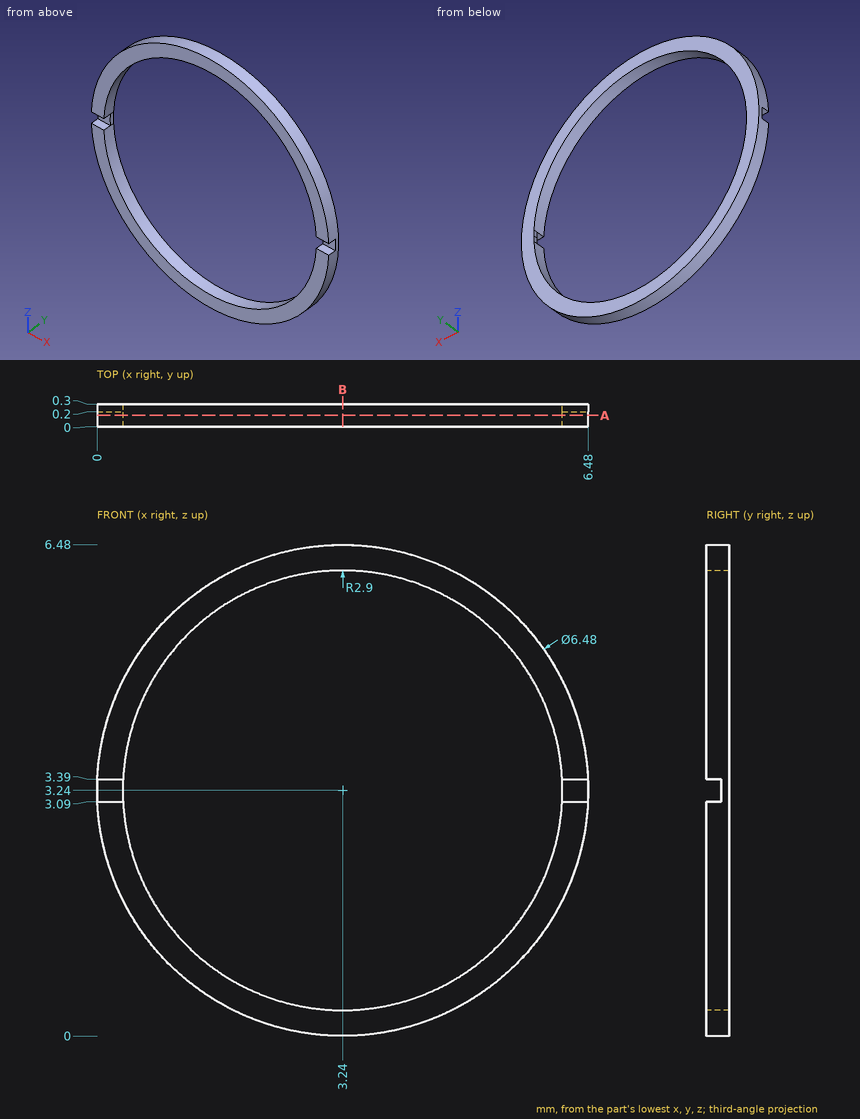
Could you check a few things on this drawing? It's one solid part, dimensions in mm from its lowest x, y, z. Round coordinates to 2 decimals unless told otherwise and drop trailing zeros. Write each loop counter-clockwise with the first axis right and the second up, starting at its lowest first coordinate (ties: lowest second). Pieces come first, ordered by that corner, then holes.
Q1. If we section it at A-A on y = 0.15: Write out the boundary of the cut face in (x, z).
Q2. If we section it at B-B on x = 3.24: Write out the boundary of the cut face in (y, z).
Q3. Please list where these lines run through material, in increasing order: probe 1 along Z at (x, y) = (4.25, 0.15); probe 2 along X at (y, z) = (0.2, 3.75); probe 3 along X at (y, z) = (0.2, 3.5).
Answer below:
1. outline: (0, 3.09) arc R3.24 ccw to (6.48, 3.09) - (6.14, 3.09) arc R2.9 cw to (0.34, 3.09) - close; (0, 3.39) - (0.34, 3.39) arc R2.9 cw to (6.14, 3.39) - (6.48, 3.39) arc R3.24 ccw to start
2. outline: (0, 0) - (0.3, 0) - (0.3, 0.34) - (0, 0.34) - close; (0, 6.14) - (0.3, 6.14) - (0.3, 6.48) - (0, 6.48) - close
3. probe 1: z = 0.16 to 0.52, 5.96 to 6.32
3. probe 2: x = 0.04 to 0.39, 6.09 to 6.44
3. probe 3: x = 0.01 to 0.35, 6.13 to 6.47
